Autodesk Inventor part; units mm, degrees
ref_plane "YZ Plane" through (0, 0, 0) normal (1, 0, 0) x (0, 1, 0)
ref_plane "XZ Plane" through (0, 0, 0) normal (0, 1, 0) x (-1, 0, 0)
ref_plane "XY Plane" through (0, 0, 0) normal (0, 0, 1) x (1, 0, 0)
sketch "Sketch1" plane through (0, 0, 0) normal (0, 0, 1) x (1, 0, 0)
  circle A0 centre (0, 0) radius 9.525
  dimension "d0" = 19.05
extrude "Extrusion1" add sketch "Sketch1" along normal blind 19.05
sketch "Sketch2" plane through (0, 0, 19.05) normal (0, 0, 1) x (1, 0, 0)
  circle A0 centre (0, 0) radius 8.1534
  circle A1 centre (0, 0) radius 4.445
  circle A2 centre (0, 0) radius 9.525
  dimension "d3" = 8.89
  dimension "d4" = 1.3716
extrude "Extrusion2" cut sketch "Sketch2" against normal blind 0.254 contours A0
hole "Hole1" at (0, 0, 0) direction (0, 0, 1) diameter 2.6416 depth 7.9375 tip angle 118
sketch "Sketch3" plane through (0, 0, 0) normal (0, 0, -1) x (-1, 0, 0)
  circle A0 centre (0, 6.4516) radius 1.778
  circle A1 centre (0, 0) radius 9.525
  circle A2 centre (0, 7.2136) radius 0.5461
  circle A3 centre (0, 5.6896) radius 0.5461
  dimension "d16" = 6.4516
  dimension "d17" = 3.556
  dimension "d20" = 1.0922
  dimension "d21" = 0.762
  dimension "d22" = 0.762
extrude "Extrusion3" add sketch "Sketch3" along normal blind 5.08 contours A0 | A2 | A3
sketch "Sketch4" plane through (0, 6.4516, -5.08) normal (0, 0, -1) x (-1, 0, 0)
  circle A0 centre (0, 0.773) radius 0.5212
  circle A1 centre (0, -0.7642) radius 0.5469
  point P0 (0, -6.4516)
extrude "Extrusion4" add sketch "Sketch4" along normal blind 3.81
properties part number "CE-075-12C"
Geometry: final body of the model. Coordinates: model frame, mm. A direction names the side the tool comes from. Give positions to 0.01 mm unless a question says otherwise; leave off trailing zeros. Order: outer loops, then holes, each group sorted by start corner. A loop starts at its lowest first (then second) coordinate and runs counter-clockwise, first axis right, second up. Notation, with made-up numbers: (79, 20) -> (124, 20) arc R27 ccw to (124, 54) -> close; hole circle Ø9 at (45, -28.75). An arc over 180 degrees is marked (long way). Put each result on its own line as item: value.
Q1. Section D-D, the plane z = 12. Return loops of the section in (x, y) (3 decimals), then the cut area to 3 significant figures.
Here are the results:
outline: circle Ø19.05 at (0, 0)
area: 285 mm^2
Q2. Section A-A, the plane z = 0.5. Return loops of the section in (x, y) (3 decimals), then the cut area to 3 significant figures.
Here are the results:
outline: circle Ø19.05 at (0, 0); hole circle Ø2.642 at (0, 0)
area: 280 mm^2
Q3. Section B-B, the plane y = -2.75. Return loops of the section in (x, z), then the cut area to 3 significant figures.
Here are the results:
outline: (-9.12, 0) -> (9.12, 0) -> (9.12, 19.05) -> (7.68, 19.05) -> (7.68, 18.8) -> (3.49, 18.8) -> (3.49, 19.05) -> (-3.49, 19.05) -> (-3.49, 18.8) -> (-7.68, 18.8) -> (-7.68, 19.05) -> (-9.12, 19.05) -> close
area: 345 mm^2
Q4. Pin query (flat end, axial travel): pin 1 (8 mm diameter, centred on x = -3, z = 10, fed in from +Y) (3 decimals); pin 2 (8 mm diameter, centred on y = -7, z = -0.5, fed in from +X); pin 3 (3 mm diameter, centred on x = 2.5, z = -3.5, fed in from +Y); pin 4 (1.5 mm diameter, centred on x = -2, y = -2, fed in from -Z). Return the tip coordinate at first contact, or that it passes through.
Here are the results:
pin 1: stops at y = 9.525
pin 2: stops at x = 9.03
pin 3: stops at y = 7.92
pin 4: stops at z = 0
Q5. Material intervals for L1, parallel to Y at x = 0, z = 19 (3 decimals); L2, parallel to Y at x = 0, z = 2.5 (3 decimals); L3, parallel to Z at x = -4.25, y = 8.25, sorted ascending.
Here are the results:
L1: y = -9.525 to -8.153, -4.445 to 4.445, 8.153 to 9.525
L2: y = -9.525 to -1.321, 1.321 to 9.525
L3: z = 0 to 19.05
Q6. Draft query along X for faces 1 (the face through (-7.559, 5.796, 9.392)), 2 (the face through (0, -2, 0)), 3 (the face through (0.8, -1.05, 4.02)). Return one class per face: released by +X, released by -X, zero draft, split by the parting line, or undercut.
Here are the results:
face 1: split by the parting line
face 2: zero draft
face 3: undercut
Q7. Reachability of faces 4 (the face through (0, 6, -8.89)), 5 (the face through (0.23, 4.69, -2.5)), 6 (the face through (4, -4, 18.796)) from +Z, -Z, +X, -X, +Y, -Y: full face, straight path, thin tool, end or side. Return the list, or none.
Here are the results:
face 4: -Z, +X, -X, +Y, -Y
face 5: -Z
face 6: +Z
Q8. Section C-C, the plane x = 2.5. Return loops of the section in (y, z), then the cut area to 3 significant figures.
Here are the results:
outline: (-9.19, 0) -> (9.19, 0) -> (9.19, 19.05) -> (7.76, 19.05) -> (7.76, 18.8) -> (3.68, 18.8) -> (3.68, 19.05) -> (-3.68, 19.05) -> (-3.68, 18.8) -> (-7.76, 18.8) -> (-7.76, 19.05) -> (-9.19, 19.05) -> close
area: 348 mm^2
